Part print with two shaded views. Sizes in mm from the minimum x, y, z corner. Give positions to 0.01 mm unless a question says otherwise; leave off trailing zeros. Write each loop counter-clockwise with the first axis right and the second up, starting at its lowest first coordinate (ties: lowest second). Pieces come first, ordered by that corner, then holes.
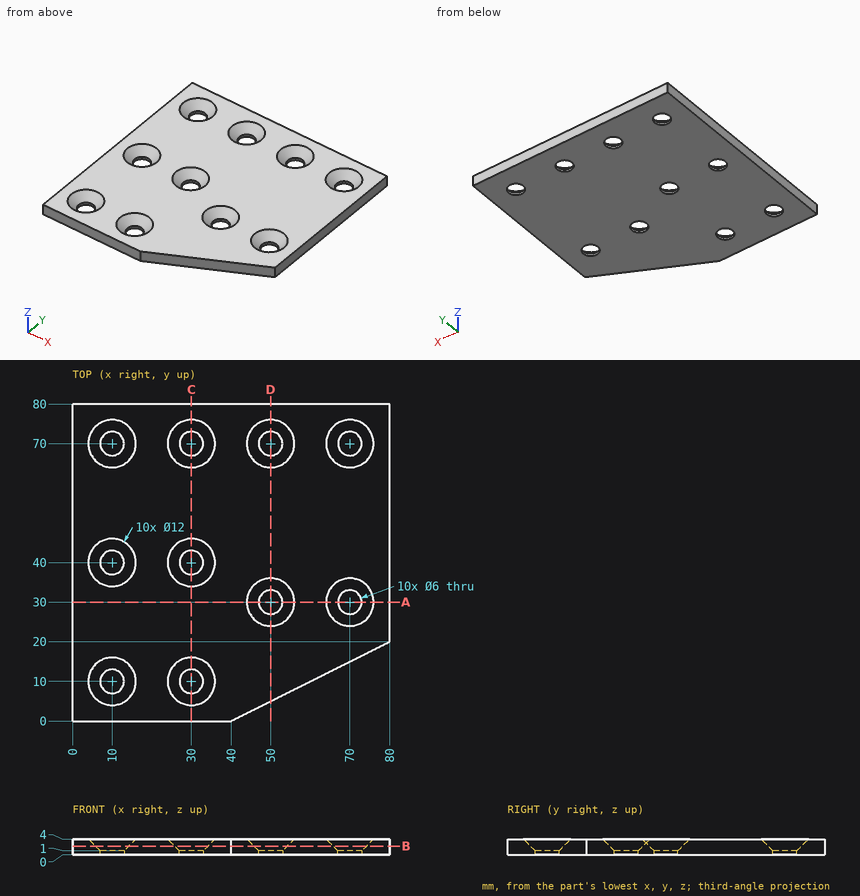
1) Saw through at A-A, the plane y = 30. Write the cut outline in (x, z), then the cut area to 3 significant figures.
Answers follow:
outline: (0, 0) - (47, 0) - (47, 1) - (44, 4) - (0, 4) - close; (53, 0) - (67, 0) - (67, 1) - (64, 4) - (56, 4) - (53, 1) - close; (73, 0) - (80, 0) - (80, 4) - (76, 4) - (73, 1) - close
area: 254 mm2
2) Saw through at C-C, the plane x = 30. Write the cut outline in (y, z), then the cut area to 3 significant figures.
Answers follow:
outline: (0, 0) - (7, 0) - (7, 1) - (4, 4) - (0, 4) - close; (13, 0) - (37, 0) - (37, 1) - (34, 4) - (16, 4) - (13, 1) - close; (43, 0) - (67, 0) - (67, 1) - (64, 4) - (46, 4) - (43, 1) - close; (73, 0) - (80, 0) - (80, 4) - (76, 4) - (73, 1) - close
area: 221 mm2
3) Saw through at D-D, the plane x = 50. Write the cut outline in (y, z).
Answers follow:
outline: (5, 0) - (27, 0) - (27, 1) - (24, 4) - (5, 4) - close; (33, 0) - (67, 0) - (67, 1) - (64, 4) - (36, 4) - (33, 1) - close; (73, 0) - (80, 0) - (80, 4) - (76, 4) - (73, 1) - close
4) Saw through at B-B, the plane z = 2.2. Count the separate pieces of the cut face and the enclosed holes in it, then the cut area to 3 significant figures.
Answers follow:
separate pieces: 1
enclosed holes: 10
area: 5,450 mm2
5) Pin check, flat tips, straight feed: pin 1 Ø9.5 at (x, y) = (30, 10) entering from +Z; pin 2 Ø7 at (x, y) = (50, 70) entering from +Z; pin 3 Ø8 at (x, y) = (30, 40) entering from +Z. Stop position of each tip, or through.
Answers follow:
pin 1: stops at z = 2.75
pin 2: stops at z = 1.5
pin 3: stops at z = 2
6) Wall check: L1, parallel to Y at x = 10, z = 0.55; L2, parallel to X at y = 5.5, z = 3.4; L3, parallel to Y at x = 50, z = 0.8. Give the ranges that are in metal, low to high.
Answers follow:
L1: y = 0 to 7, 13 to 37, 43 to 67, 73 to 80
L2: x = 0 to 7.02, 12.98 to 27.02, 32.98 to 51
L3: y = 5 to 27, 33 to 67, 73 to 80
